```python
from build123d import *

# Parameters (mm, degrees)
BOSS_EXTRUDE1_DEPTH = 6.35
CUT_EXTRUDE1_DEPTH  = 6.35
LPATTERN1_COUNT     = 2
LPATTERN1_PITCH     = 30
SKETCH4_W           = 6.35
SKETCH4_H           = 13
BOSS_EXTRUDE2_DEPTH = 6.35
SKETCH5_R           = 6.75
CUT_EXTRUDE2_DEPTH  = 82.536157623


with BuildPart() as part:
    # Sketch2 → Boss-Extrude1 (new body)
    with BuildSketch(Plane.XY):
        with BuildLine():
            Line((-25, 0), (-25, -75))
            Line((-25, -75), (25, -75))
            Line((25, -75), (25, 0))
            ThreePointArc((25, 0), (0, 25), (-25, 0))
        make_face()
    extrude(amount=BOSS_EXTRUDE1_DEPTH)

    # Sketch3 → Cut-Extrude1 (cut)
    with BuildSketch(Plane.XY.offset(6.35)):
        Polygon((-12.3, -67.54), (-16.999, -67.54), (-16.999, -70.4991), (-20.301, -70.4991), (-20.301, -67.54), (-25, -67.54), (-25, -62.46), (-20.301, -62.46), (-20.301, -59.5009), (-16.999, -59.5009), (-16.999, -62.46), (-12.3, -62.46), align=None)
    cut_extrude1 = extrude(amount=-CUT_EXTRUDE1_DEPTH, mode=Mode.SUBTRACT)

    # LPattern1: Cut-Extrude1 ×2
    with Locations(*[(0, i * LPATTERN1_PITCH, 0) for i in range(1, LPATTERN1_COUNT)]):
        add(cut_extrude1, mode=Mode.SUBTRACT)

    # Sketch4 → Boss-Extrude2 (add)
    with BuildSketch(Plane.XY.offset(6.35)):
        with Locations((-28.175, -50)):
            Rectangle(SKETCH4_W, SKETCH4_H)
    extrude(amount=-BOSS_EXTRUDE2_DEPTH)

    # Sketch5 → Cut-Extrude2 (cut, through all)
    with BuildSketch(Plane.XY.offset(6.35)):
        Circle(SKETCH5_R)
    extrude(amount=-CUT_EXTRUDE2_DEPTH, mode=Mode.SUBTRACT)


solid = part.part
```
Check sheet for the modelled part. Datum: model origin and axes. Units: mm. A direction names the side the tool comes from. Coordinates: 2 decimals unless noted, no trailing zeros. Write each loop counter-clockwise with the first axis right and the second up, starting at its lowest first coordinate (ties: lowest second). Pieces come first, ordered by that corner, then holes. Notation, with made-up numbers: M 18.25,-17 L 29.25,-17 A27 ccw 29.25,15 Z; hole C 88.25,30.25 d3. An arc over 180 degrees is marked long. Write item = value, one per line. Start each with the question number.
1. Mould release check, pull along X, two halves, no side actions. Record for faces 1 (the flat face through (-25, -40, 3)), 2 (the flat face through (-15, -67.54, 3)), 3 (the cylindrical face through (-1.46, -6.59, 3.22)), 4 (the flat face through (-16.999, -69, 3)): pulls with the +X half, pulls with the -X half, needs draft (parallel to the pull), parting line crosses it, or undercut.
2. Thickness scan on probe 1 along Y at (x, z) = (-18, 0.5); probe 2 along Y at (x, z) = (0, 1.75); probe 3 along X at (y, z) = (-62, 0.75). Record the ranges inside material, lowest first.
3. Sectioned sample at C-C (y = -3). Record the cut outline in (x, z).
4. Tool access check on faces 5 (the flat face through (-20.301, -69, 3)), 6 (the flat face through (-28, -56.5, 3)), 7 (the flat face through (-23, -32.46, 3)). Record the directions out of +Z, -Z, +X, -X, +Y, -Y that give a thin tool (end or side, any length) a straight path to the whole face; none if there is none.
5. Sectioned sample at A-A (x = 0). Record the cut outline in (y, z), then the cut area to 3 significant figures.
6. Sectioned sample at D-D (y = 15). Record the cut outline in (x, z), then the cut area to 3 significant figures.
7. Go/stop test with flat-tipped pins: pin 1 (2.5 mm diameter, centred on y = -65.5, z = 3, fed in from -X); pin 2 (3.5 mm diameter, centred on x = -19, z = 3, fed in from +Y); pin 3 (1.9 mm diameter, centred on x = -29, z = 4, fed in from +Y). Record where each tip stops, or that it passes through.
The answers:
q1.face_1 = pulls with the -X half
q1.face_2 = needs draft
q1.face_3 = undercut
q1.face_4 = undercut
q2.probe_1 = -75 to -70.5, -59.5 to -40.5, -29.5 to 17.35
q2.probe_2 = -75 to -6.75, 6.75 to 25
q2.probe_3 = -25 to -20.3, -17 to 25
q3.outline = M -25,0 L -6.05,0 L -6.05,6.35 L -25,6.35 Z; M 6.05,0 L 25,0 L 25,6.35 L 6.05,6.35 Z
q4.face_5 = +Z, -Z
q4.face_6 = +Z, -Z, -X, -Y
q4.face_7 = +Z, -Z, -X
q5.outline = M -75,0 L -6.75,0 L -6.75,6.35 L -75,6.35 Z; M 6.75,0 L 25,0 L 25,6.35 L 6.75,6.35 Z
q5.area = 549 mm²
q6.outline = M -20,0 L 20,0 L 20,6.35 L -20,6.35 Z
q6.area = 254 mm²
q7.pin_1 = -12.3
q7.pin_2 = 18.1
q7.pin_3 = -43.5
